from build123d import *

# Parameters (mm, degrees)
SKETCH2_R               = 6.002734375
SKETCH2_R_2             = 3.175
EXTRUDE1_DEPTH          = 11.90625
SKETCH3_R               = 1.7859375
EXTRUDE2_DEPTH          = 3.96875
CUT_EXTRUDE2_DEPTH      = 12.7
CHAMFER1_SIZE           = 0.381
CUT_EXTRUDE3_START      = -3.818600123
CUT_EXTRUDE3_OUTLINE_R  = 1.7859375
CUT_EXTRUDE3_DEPTH      = 3.818600123
CUT_EXTRUDE4_DEPTH      = 25.4
CUT_EXTRUDE4_DEPTH_BACK = 25.4
SKETCH7_W               = 25.086219796
SKETCH7_H               = 3.328995852


with BuildPart() as part:
    # Sketch2 → Extrude1 (new body)
    with BuildSketch(Plane.XY):
        Circle(SKETCH2_R)
        Circle(SKETCH2_R_2, mode=Mode.SUBTRACT)
    extrude(amount=-EXTRUDE1_DEPTH)

    # Sketch3 → Extrude2 (add)
    with BuildSketch(Plane.XY):
        with BuildLine():
            Line((-10.196981534, -4.739465365), (-2.227911932, -7.203987355))
            ThreePointArc((-2.227911932, -7.203987355), (0, -7.540625), (2.227911932, -7.203987355))
            Line((2.227911932, -7.203987355), (10.196981534, -4.739465365))
            ThreePointArc((10.196981534, -4.739465365), (13.6921875, 0), (10.196981534, 4.739465365))
            Line((10.196981534, 4.739465365), (2.227911932, 7.203987355))
            ThreePointArc((2.227911932, 7.203987355), (0, 7.540625), (-2.227911932, 7.203987355))
            Line((-2.227911932, 7.203987355), (-10.196981534, 4.739465365))
            ThreePointArc((-10.196981534, 4.739465365), (-13.6921875, 0), (-10.196981534, -4.739465365))
        make_face()
        with Locations((8.73125, 0)):
            Circle(SKETCH3_R, mode=Mode.SUBTRACT)
        with Locations((-8.73125, 0)):
            Circle(SKETCH3_R, mode=Mode.SUBTRACT)
    extrude(amount=-EXTRUDE2_DEPTH)

    # Cut-Extrude1 cone 1 section (through the dimple's axis) → Cut-Extrude1 (revolve, cut)
    with BuildSketch(Plane(origin=(8.73125, 0, 0), x_dir=(0, -1, 0), z_dir=(1, 0, 0))):
        Polygon((0, 0), (3.571875, 0), (0, 2.997158995), align=None)
    revolve(axis=Axis((8.73125, 0, 0), (0, 0, -1)), mode=Mode.SUBTRACT)

    # Cut-Extrude1 cone 2 section (through the dimple's axis) → Cut-Extrude1 cone 2 (revolve, cut)
    with BuildSketch(Plane(origin=(-8.73125, 0, 0), x_dir=(0, -1, 0), z_dir=(1, 0, 0))):
        Polygon((0, 0), (3.571875, 0), (0, 2.997158995), align=None)
    revolve(axis=Axis((-8.73125, 0, 0), (0, 0, -1)), mode=Mode.SUBTRACT)

    # Sketch5 → Cut-Extrude2 (cut, symmetric)
    with BuildSketch(Plane(origin=(0, 0, 0), x_dir=(1, 0, 0), z_dir=(0, 1, 0))):
        with BuildLine():
            Line((13.6921875, 0.9921875), (13.6921875, -0.635))
            Line((13.6921875, -0.635), (-13.6921875, -0.635))
            Line((-13.6921875, -0.635), (-13.6921875, 0.9921875))
            ThreePointArc((-13.6921875, 0.9921875), (0, 0), (13.6921875, 0.9921875))
        make_face()
    extrude(amount=CUT_EXTRUDE2_DEPTH, both=True, mode=Mode.SUBTRACT)

    # Chamfer1
    chamfer1_edges = [part.edges().sort_by_distance(p)[0] for p in [
        (-6.002734375, 0, -11.90625),
        (-3.175, 0, -11.90625),
    ]]
    chamfer(chamfer1_edges, length=CHAMFER1_SIZE)

    # Cut-Extrude3: read off the stored shape, not the designer's step
    # Cut-Extrude3 outline → Cut-Extrude3 (cut)
    # profile 1 of 2: a face of its own
    with BuildSketch(Plane(origin=(0, 0, -3.96875), x_dir=(-1, 0, 0), z_dir=(0, 0, -1)).offset(CUT_EXTRUDE3_START)):
        with BuildLine():
            ThreePointArc((-12.543109898, 3.175), (-13.6921875, 0), (-12.543109898, -3.175))
            Line((-12.543109898, -3.175), (-8.73125, -3.175))
            ThreePointArc((-8.73125, -3.175), (-5.55625, 0), (-8.73125, 3.175))
            Line((-8.73125, 3.175), (-12.543109898, 3.175))
        make_face()
        with Locations((-8.73125, 0)):
            Circle(CUT_EXTRUDE3_OUTLINE_R, mode=Mode.SUBTRACT)
    # profile 2 of 2: a face of its own
    with BuildSketch(Plane(origin=(0, 0, -3.96875), x_dir=(-1, 0, 0), z_dir=(0, 0, -1)).offset(CUT_EXTRUDE3_START)):
        with BuildLine():
            ThreePointArc((8.73125, 3.175), (5.55625, 0), (8.73125, -3.175))
            Line((8.73125, -3.175), (12.543109898, -3.175))
            ThreePointArc((12.543109898, -3.175), (13.6921875, 0), (12.543109898, 3.175))
            Line((12.543109898, 3.175), (8.73125, 3.175))
        make_face()
        with Locations((8.73125, 0)):
            Circle(CUT_EXTRUDE3_OUTLINE_R, mode=Mode.SUBTRACT)
    extrude(amount=CUT_EXTRUDE3_DEPTH, mode=Mode.SUBTRACT)

    # Cut-Extrude3 2 outline → Cut-Extrude3 2 (revolve, cut)
    with BuildSketch(Plane(origin=(8.73125, 0, 0), x_dir=(1, 0, 0), z_dir=(0, -1, 0))):
        Polygon((2.728509965, -3.968749996), (2.728509965, -9.072154448), (3.175, -3.968749996), align=None)
    revolve(axis=Axis((8.73125, 0, 0), (0, 0, 1)), mode=Mode.SUBTRACT)

    # Cut-Extrude3 3 outline → Cut-Extrude3 3 (revolve, cut)
    with BuildSketch(Plane(origin=(-8.73125, 0, 0), x_dir=(1, 0, 0), z_dir=(0, -1, 0))):
        Polygon((2.728515625, -3.968749996), (2.728515625, -9.07208976), (3.175, -3.968749996), align=None)
    revolve(axis=Axis((-8.73125, 0, 0), (0, 0, 1)), mode=Mode.SUBTRACT)

    # Sketch7 → Cut-Extrude4 (cut, two sides: drawn at the far end of the back side and taken through both)
    with BuildSketch(Plane(origin=(0, 0, 0), x_dir=(1, 0, 0), z_dir=(0, 1, 0)).offset(-CUT_EXTRUDE4_DEPTH_BACK)):
        with Locations((0, -0.870747926)):
            Rectangle(SKETCH7_W, SKETCH7_H)
    extrude(amount=CUT_EXTRUDE4_DEPTH + CUT_EXTRUDE4_DEPTH_BACK, mode=Mode.SUBTRACT)


solid = part.part
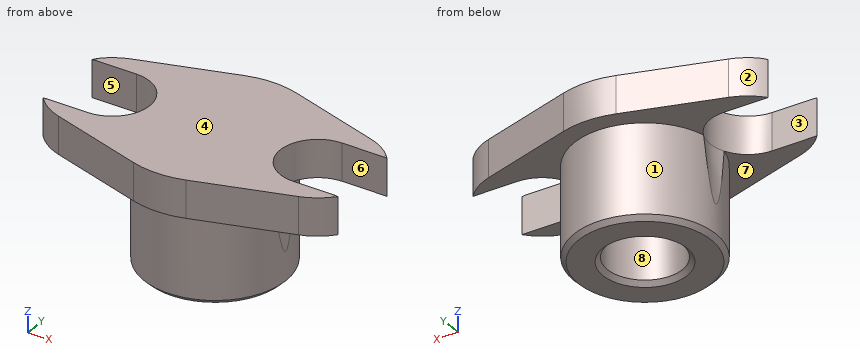
Read the model definition and answer for the solid it produces. Units are mm, in the model's axes. Face numbers are marked on the shaded views. A direction names the side the tool comes from. Give positions to 0.01 mm unless a question says otherwise; leave off trailing zeros. Loops run counter-clockwise (first coordinate to the right, second up) from the corner with the lowest first, then second, coordinate; pieces in that order, holes last. Notation, with made-up numbers: M 10.5,-35 L 55.5,-35 A21 cw 55.5,-12 Z; hole C -26,47.5 d4. An arc over 180 degrees is marked long. Write each question's results on one line, items separated by ' | '.
1. A tool of negligible diameter and unlimited length cuts with its end or side. For the marked faces 5, 6, 7 and 8, from which of +Z, -Z, +X, -X, +Y, -Y can it reach the whole face along a straight path? Write none if from no direction.
Values:
face 5: +Z, -Z, -X | face 6: +Z, -Z, +X | face 7: -Z, -Y | face 8: -Z
2. Straight lines are drawn through the part: line 1 (Y direction, x = 0, z = -5.5) (3 decimals); line 2 (Z direction, x = -5.25, y = -5.25); line 3 (Y direction, x = 0.5, z = -5.5). For each, find the intervals that lie inside material, in ascending order. Write a range as [from, to].
Values:
line 1: y = [-6.003, -3.175], [3.175, 6.003] | line 2: z = [-3.97, -0.79] | line 3: y = [-5.98, -3.14], [3.14, 5.98]
3. Section A-A on x = 0 is taken. Give the vertices of the cut face in (y, z) (3 decimals), plus the area to 3 significant figures.
Values:
outline: M -7.541,-3.969 L -6.003,-3.969 L -6.003,-11.525 L -5.622,-11.906 L -3.556,-11.906 L -3.175,-11.525 L -3.175,-3.969 L 3.175,-3.969 L 3.175,-11.525 L 3.556,-11.906 L 5.622,-11.906 L 6.003,-11.525 L 6.003,-3.969 L 7.541,-3.969 L 7.541,-0.794 L -7.541,-0.794 Z | area: 92.5 mm^2
4. The mould has two halves that part along Y. Classify the marked faces 1, 2, 3 and 4: pulls with the +Y half, pulls with the -Y half, needs draft (parallel to the pull), parting line crosses it, or undercut.
Values:
face 1: parting line crosses it | face 2: pulls with the +Y half | face 3: undercut | face 4: needs draft
5. Section D-D on y = -6.5 is taken. Give the vertices of the cut face in (x, z).
Values:
outline: M -4.5,-3.97 L 4.5,-3.97 L 4.5,-0.79 L -4.5,-0.79 Z
6. Given pin 1 (3.5 mm diameter, centred on x = -11, z = -2.5, fed in from -Y); pin 2 (1 mm diameter, centred on y = -2, z = -9, fed in from +X); pin 3 (3 mm diameter, centred on x = 5, z = -2.5, fed in from +Y), each flat-ended and moving along its own axis, determine where each tip first touches the part or whether it passes through.
Values:
pin 1: stops at y = -5.03 | pin 2: stops at x = 5.81 | pin 3: stops at y = 6.81
7. Section B-B on y = 0 is taken. Give the vertices of the cut face in (x, z) (3 decimals).
Values:
outline: M -6.003,-11.525 L -5.622,-11.906 L -3.556,-11.906 L -3.175,-11.525 L -3.175,-3.969 L 3.175,-3.969 L 3.175,-11.525 L 3.556,-11.906 L 5.622,-11.906 L 6.003,-11.525 L 6.003,-9.072 L 5.556,-3.969 L 5.556,-0.794 L -5.556,-0.794 L -5.556,-3.969 L -6.003,-9.072 Z
8. Section C-C on z = -8 is taken. Give the vertices of the cut face in (x, y) (3 decimals).
Values:
outline: M -5.973,-0.598 A6.003 ccw 5.973,-0.598 A2.822 cw 5.973,0.598 A6.003 ccw -5.973,0.598 A2.822 cw Z; hole C 0,0 d6.35
